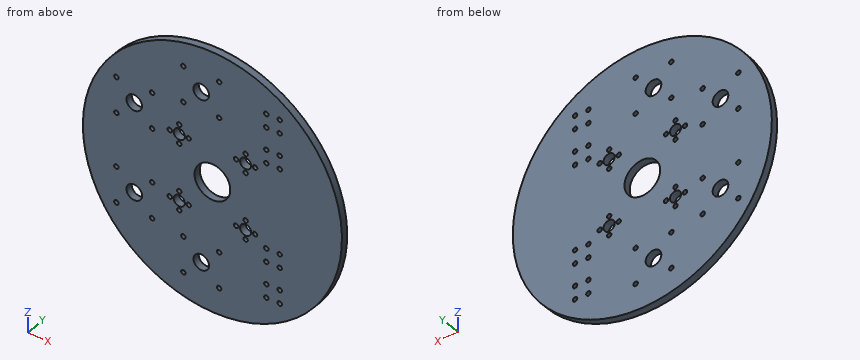
Autodesk Inventor part; units mm, degrees
ref_plane "YZ Plane" through (0, 0, 0) normal (1, 0, 0) x (0, 1, 0)
ref_plane "XZ Plane" through (0, 0, 0) normal (0, 1, 0) x (-1, 0, 0)
ref_plane "XY Plane" through (0, 0, 0) normal (0, 0, 1) x (1, 0, 0)
sketch "Sketch1" plane through (0, 0, 0) normal (0, 1, 0) x (-1, 0, 0)
  circle A0 centre (0, 0) radius 116
  dimension "d0" = 232
extrude "Extrusion1" add sketch "Sketch1" along normal mid plane 6.35
sketch "Sketch2" plane through (0, 3.175, 0) normal (0, 1, 0) x (1, 0, 0)
  circle A0 centre (-42, 0) radius 5
  circle A1 centre (-36, 6) radius 2
  circle A2 centre (-48, 6) radius 2
  circle A3 centre (-48, -6) radius 2
  circle A4 centre (-36, -6) radius 2
  circle A5 centre (0, -42) radius 5
  circle A6 centre (-6, -36) radius 2
  circle A7 centre (-6, -48) radius 2
  circle A8 centre (6, -48) radius 2
  circle A9 centre (6, -36) radius 2
  circle A10 centre (42, 0) radius 5
  circle A11 centre (36, -6) radius 2
  circle A12 centre (48, -6) radius 2
  circle A13 centre (48, 6) radius 2
  circle A14 centre (36, 6) radius 2
  circle A15 centre (0, 42) radius 5
  circle A16 centre (6, 36) radius 2
  circle A17 centre (6, 48) radius 2
  circle A18 centre (-6, 48) radius 2
  circle A19 centre (-6, 36) radius 2
  point P0 (0, 0)
  dimension "d3" = 10
  dimension "d4" = 42
  dimension "d5" = 4
  dimension "d6" = 6
  dimension "d7" = 6
  dimension "d10" = 360
  dimension "d14" = 360
extrude "Extrusion2" cut sketch "Sketch2" against normal through all
sketch "Sketch3" plane through (0, 3.175, 0) normal (0, 1, 0) x (1, 0, 0)
  circle A0 centre (0, 0) radius 16
  dimension "d18" = 32
extrude "Extrusion3" cut sketch "Sketch3" against normal through all
move or copy body "Move Body1" bodies to move or copy 1 copy no rotation origin (0, 0, 0) rotation axis (0, 1, 0) rotation angle -45
sketch "Sketch4" plane through (0, 3.175, 0) normal (0, 1, 0) x (1, 0, 0)
  circle A0 centre (0, 0) radius 16 construction
  line L0 (-16, 0) -> (16, 0) construction
  line L1 (0, 16) -> (0, -16) construction
  circle A1 centre (54.2525, -76) radius 2.5 construction
  circle A2 centre (48.2525, -82) radius 2
  circle A3 centre (60.2525, -82) radius 2
  circle A4 centre (60.2525, -70) radius 2
  circle A5 centre (48.2525, -70) radius 2
  line L2 (54.2525, -76) -> (54.2525, -44) construction
  circle A6 centre (54.2525, -44) radius 2.5 construction
  circle A7 centre (48.2525, -50) radius 2
  circle A8 centre (60.2525, -50) radius 2
  circle A9 centre (60.2525, -38) radius 2
  circle A10 centre (48.2525, -38) radius 2
  circle A11 centre (54.2525, 76) radius 2.5 construction
  circle A12 centre (48.2525, 82) radius 2
  circle A13 centre (60.2525, 82) radius 2
  circle A14 centre (60.2525, 70) radius 2
  circle A15 centre (48.2525, 70) radius 2
  line L3 (54.2525, 76) -> (54.2525, 44) construction
  circle A16 centre (54.2525, 44) radius 2.5 construction
  circle A17 centre (48.2525, 50) radius 2
  circle A18 centre (60.2525, 50) radius 2
  circle A19 centre (60.2525, 38) radius 2
  circle A20 centre (48.2525, 38) radius 2
  dimension "d35" = 5
  dimension "d37" = 4
  dimension "d38" = 6
  dimension "d39" = 6
  dimension "d42" = 360
  dimension "d44" = 32
  dimension "d45" = 5
  dimension "d46" = 4
  dimension "d47" = 6
  dimension "d48" = 6
  dimension "d51" = 360
  dimension "d78" = 76
extrude "Extrusion4" cut sketch "Sketch4" against normal through all
sketch "Sketch5" plane through (0, 3.175, 0) normal (0, 1, 0) x (1, 0, 0)
  circle A0 centre (-10, 76) radius 7
  circle A1 centre (-26, 92) radius 2
  circle A2 centre (-26, 60) radius 2
  circle A3 centre (6, 60) radius 2
  circle A4 centre (6, 92) radius 2
  circle A5 centre (0, 0) radius 16 construction
  line L0 (-16, 0) -> (16, 0) construction
  circle A6 centre (-10, -76) radius 7
  circle A7 centre (-26, -92) radius 2
  circle A8 centre (-26, -60) radius 2
  circle A9 centre (6, -60) radius 2
  circle A10 centre (6, -92) radius 2
  line L1 (0, 16) -> (0, -16) construction
  circle A11 centre (-70, 40) radius 7
  circle A12 centre (-54, 56) radius 2
  circle A13 centre (-86, 56) radius 2
  circle A14 centre (-86, 24) radius 2
  circle A15 centre (-54, 24) radius 2
  circle A16 centre (-70, -40) radius 7
  circle A17 centre (-54, -56) radius 2
  circle A18 centre (-86, -56) radius 2
  circle A19 centre (-86, -24) radius 2
  circle A20 centre (-54, -24) radius 2
  dimension "d55" = 14
  dimension "d56" = 10
  dimension "d57" = 76
  dimension "d58" = 4
  dimension "d59" = 16
  dimension "d60" = 16
  dimension "d63" = 360
  dimension "d67" = 14
  dimension "d68" = 4
  dimension "d69" = 16
  dimension "d70" = 16
  dimension "d71" = 40
  dimension "d75" = 360
  dimension "d79" = 70
extrude "Extrusion5" cut sketch "Sketch5" against normal through all
properties part number "TurnTableTop"
Design review of the part built by this model. Coordinates are the model's own, in mm. Coordinates: 2 decimals unless noted, no trailing zeros. Order: outer loops, then holes, each group sorted by start corner. A loop starts at its lowest first (then second) coordinate and runs counter-clockwise, first axis right, second up. Notation, with made-up numbers: (17.5, -5) -> (75.5, -5) arc R12 ccw to (75.5, 8) -> close; hole circle Ø1 at (33, 85). An arc over 180 degrees is marked (long way). One line per item, written item: value. Start each with the question number.
Q1. Take a section at D-D, the plane z = 87. State the section outline as (x, y) points (3 decimals).
Q2. Take a section at A-A, the plane z = 0.5. State the section outline as (x, y) points (3 decimals).
Q3. Insertion check: pin 1 Ø3 at (x, z) = (-26, 92) entering from +Y; pin 2 Ø1.5 at (x, y) = (67, 0) entering from +Z; pin 3 Ø1.5 at (y, z) = (-1, -43) entering from -X; pin 4 Ø3 at (y, z) = (2, 21.5) entering from -X. Each pin has a flat end and moves straight along its axis. Give the tip position at first contact, or say it passes through.
Q4. Take a section at C-C, the plane x = -97. State the section outline as (y, z) points (3 decimals).
Q5. Take a section at B-B, the plane y = 1.75. Give the number of separate pieces and of enclosed holes in the cut face, then the cut area to 3 significant figures.
Q6. For probe 1 along Z at (x, y) = (-86, -0.75); probe 2 along X at (y, z) = (-0.25, 38); probe 3 along Z at (x, y) = (-19.5, -0.5), list the stretches that pass through material, from the lowest coordinate up.
Values follow:
1. outline: (-76.727, -3.175) -> (76.727, -3.175) -> (76.727, 3.175) -> (-76.727, 3.175) -> close
2. outline: (-115.999, -3.175) -> (-15.992, -3.175) -> (-15.992, 3.175) -> (-115.999, 3.175) -> close; (15.992, -3.175) -> (115.999, -3.175) -> (115.999, 3.175) -> (15.992, 3.175) -> close
3. pin 1: passes through
3. pin 2: stops at z = 95.22
3. pin 3: stops at x = -108.03
3. pin 4: stops at x = -114.26
4. outline: (-3.175, -63.616) -> (3.175, -63.616) -> (3.175, 63.616) -> (-3.175, 63.616) -> close
5. separate pieces: 1
5. enclosed holes: 57
5. area: 39,900 mm2
6. probe 1: z = -77.85 to -58, -54 to -26, -22 to 22, 26 to 54, 58 to 77.85
6. probe 2: x = -109.6 to -76.71, -63.29 to -31.69, -27.71 to 27.71, 31.69 to 46.25, 50.25 to 58.25, 62.25 to 109.6
6. probe 3: z = -114.35 to -30.73, -28.67 to 28.67, 30.73 to 114.35
